Here's how the part is built. I have some questions about the finished solid (model axes, mm). Round coordinates to 2 decimals unless told otherwise and drop trailing zeros. Loops run counter-clockwise (first coordinate to the right, second up) from the corner with the lowest first, then second, coordinate; pieces in that order, holes last. Notation, with made-up numbers: (-20, 80.25) -> (35, 80.25) arc R12 ccw to (35, 89.25) -> close; hole circle Ø9 at (45, 55). An arc over 180 degrees is marked (long way). Use one line per item in the form item = value. Start each with the question number.
Item 1: If we section it at A-A (y = 32): Write out the boundary of the cut face in (x, z), then the cut area to 3 significant figures.
Item 2: If we section it at C-C (x = 63.5): Write out the boundary of the cut face in (y, z).
Item 3: Thinking about a two-plate mould opening in X: for faces 1 (the face through (-124.88, 5.5, 1.48)), 2 (the face through (83.11, -82.77, 1.64)), 3 (the face through (-112, -9, 0)), which applies, released by +X, released by -X, zero draft, split by the parting line, or undercut?
Item 4: I'm going to push flat-ended pins straight in: pin 1 Ø2.5 at (x, y) = (-81.67, -81.67) entering from +Z; pin 2 Ø4.5 at (x, y) = (-115.5, 0) entering from -Z; pin 3 Ø4 at (x, y) = (81.67, 81.67) entering from +Z; pin 4 Ø1 at (y, z) = (63.5, 2.5) entering from -X. Where does each tip first touch, or does it pass through?
Item 5: If I drill on L1, parallel to Y at x = 0, z = 2.1; L2, parallel to X at y = -80.5, z = 2.5; L3, parallel to Y at x = 115.5, z = 2.25, over which ranges is the centre line in solid material (lowest first)? Write a range as [from, to].
Item 6: If we section it at B-B (z = 2.5): State how many separate pieces and enclosed holes the cut face has, then the cut area to 3 significant figures.
```python
from build123d import *

# Parameters (mm, degrees)
SKETCH1_R           = 125
SKETCH1_R_2         = 112
BOSS_EXTRUDE1_DEPTH = 3
CIRPATTERN1_COUNT   = 8


with BuildPart() as part:
    # Sketch1 → Boss-Extrude1 (new body)
    with BuildSketch(Plane.XY):
        Circle(SKETCH1_R)
        Circle(SKETCH1_R_2, mode=Mode.SUBTRACT)
    extrude(amount=BOSS_EXTRUDE1_DEPTH)

    # Sketch3 → CSK for M3 Countersunk Flat Head Screw1 (revolve, cut)
    with BuildSketch(Plane.YZ.offset(-115.5)):
        Polygon((0, 0), (0, 3), (1.7, 3), (1.7, 1.75), (3.45, 0), align=None)
    csk_for_m3_countersunk_flat_head_screw1 = revolve(axis=Axis((-115.5, 0, -6.35), (0, 0, 1)), mode=Mode.SUBTRACT)

    # CirPattern1: CSK for M3 Countersunk Flat Head Screw1 ×8 about axis
    cirpattern1_axis = Axis((0, 0, 0), (0, 0, 1))
    for i in range(1, CIRPATTERN1_COUNT):
        add(csk_for_m3_countersunk_flat_head_screw1.rotate(cirpattern1_axis, i * 360 / CIRPATTERN1_COUNT), mode=Mode.SUBTRACT)


solid = part.part
```
Values found:
q1.outline = (-120.83, 0) -> (-107.33, 0) -> (-107.33, 3) -> (-120.83, 3) -> close; (107.33, 0) -> (120.83, 0) -> (120.83, 3) -> (107.33, 3) -> close
q1.area = 81.0 mm2
q2.outline = (-107.67, 0) -> (-92.26, 0) -> (-92.26, 3) -> (-107.67, 3) -> close; (92.26, 0) -> (107.67, 0) -> (107.67, 3) -> (92.26, 3) -> close
q3.face_1 = split by the parting line
q3.face_2 = undercut
q3.face_3 = zero draft
q4.pin_1 = through
q4.pin_2 = 1.2
q4.pin_3 = 3
q4.pin_4 = -107.96
q5.L1 = [-125, -117.2], [-113.8, -112], [112, 113.8], [117.2, 125]
q5.L2 = [-95.63, -82.9], [-80.44, -77.87], [77.87, 80.44], [82.9, 95.63]
q5.L3 = [-47.8, -1.7], [1.7, 47.8]
q6.separate_pieces = 1
q6.enclosed_holes = 9
q6.area = 9,610 mm2
